Read the model definition and answer for the solid it produces. Units are mm, in the model's axes. Face numbers are marked on the shaded views. A direction names the side the tool comes from. Coordinates: 2 decimals unless noted, no trailing zeros. Loops run counter-clockwise (first coordinate to the right, second up) from the corner with the lowest first, then second, coordinate; pieces in that order, holes last. Notation, with made-up numbers: (25, 86.5) -> (41, 86.5) arc R23 cw to (41, 104.5) -> close; hole circle Ø4 at (45.5, 65). An arc over 180 degrees is marked (long way). Answer in a Markdown table with one row per item.
```python
from build123d import *

# Parameters (mm, degrees)
F0_W           = 60
F0_H           = 15
F1_DEPTH       = 7.1374
F3_D           = 3.4544
F4_D           = 4.5
F4_CBORE_D     = 7
F4_CBORE_DEPTH = 4.2
F5_SIZE        = 0.762


with BuildPart() as f1:
    # F0 (on Top) → F1 (new body)
    with BuildSketch(Plane.XY):
        Rectangle(F0_W, F0_H)
    extrude(amount=F1_DEPTH)

    # F3 (through all)
    with Locations(Plane.XY.offset(7.1374)):
        with Locations((-15, 1.76), (15, 1.76)):
            Hole(F3_D / 2)

    # F4 (through all)
    with Locations(Plane.XY.offset(7.1374)):
        with Locations((-15, -4.24), (15, -4.24)):
            CounterBoreHole(F4_D / 2, F4_CBORE_D / 2, F4_CBORE_DEPTH)

    # F5
    f5_edges = [f1.edges().sort_by_distance(p)[0] for p in [
        (0, -7.5, 7.1374),
        (-30, 0, 7.1374),
        (0, 7.5, 7.1374),
        (30, 0, 7.1374),
        (30, -7.5, 3.5687),
        (30, 7.5, 3.5687),
        (30, 0, 0),
        (0, 7.5, 0),
        (-30, 7.5, 3.5687),
        (0, -7.5, 0),
        (-30, -7.5, 3.5687),
        (-30, 0, 0),
        (23.136867, -7.5, 7.1374),
        (-23.136867, -7.5, 7.1374),
    ]]
    chamfer(f5_edges, length=F5_SIZE)


solid = f1.part
```
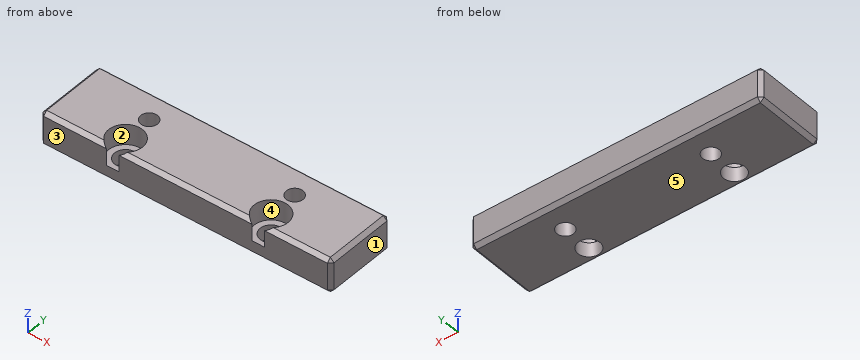
1. A cutting plane is placed at C-C on z = 1.5. Give the vertices of the cut face in (x, y).
A:
| item | result |
|---|---|
| outline | (-30, -6.74) -> (-29.24, -7.5) -> (29.24, -7.5) -> (30, -6.74) -> (30, 6.74) -> (29.24, 7.5) -> (-29.24, 7.5) -> (-30, 6.74) -> close; hole circle Ø4.5 at (-15, -4.24); hole circle Ø3.45 at (-15, 1.76); hole circle Ø4.5 at (15, -4.24); hole circle Ø3.45 at (15, 1.76) |
2. A tool of negligible diameter and unlimited length cuts with its end or side. For the marked faces 4 and 5, from which of +Z, -Z, +X, -X, +Y, -Y can it reach the whole face along a straight path? Write none if from no direction.
A:
| item | result |
|---|---|
| face 4 | +Z |
| face 5 | -Z, +X, -X, +Y, -Y |
3. A cutting plane is placed at B-B on y = 1.76. Give the vertices of the cut face in (x, z).
A:
| item | result |
|---|---|
| outline | (-30, 0.76) -> (-29.24, 0) -> (-16.73, 0) -> (-16.73, 7.14) -> (-29.24, 7.14) -> (-30, 6.38) -> close; (-13.27, 0) -> (13.27, 0) -> (13.27, 7.14) -> (-13.27, 7.14) -> close; (16.73, 0) -> (29.24, 0) -> (30, 0.76) -> (30, 6.38) -> (29.24, 7.14) -> (16.73, 7.14) -> close |
4. Given pin 1 Ø6.5 at (x, y) = (15, -4.24) entering from +Z, flat-ended and moving along its own axis, determine where the tip first touches the part or whether it passes through.
A:
| item | result |
|---|---|
| pin 1 | stops at z = 2.94 |
5. A cutting plane is placed at D-D on z = 3.75. Give the vertices of the cut face in (x, y), and give its area (3 significant figures).
A:
| item | result |
|---|---|
| outline | (-30, -6.74) -> (-29.24, -7.5) -> (-16.27, -7.5) arc R3.5 cw (long way) to (-13.73, -7.5) -> (13.73, -7.5) arc R3.5 cw (long way) to (16.27, -7.5) -> (29.24, -7.5) -> (30, -6.74) -> (30, 6.74) -> (29.24, 7.5) -> (-29.24, 7.5) -> (-30, 6.74) -> close; hole circle Ø3.45 at (-15, 1.76); hole circle Ø3.45 at (15, 1.76) |
| area | 804 mm2 |
6. Find the intervals of material crossed by probe 1 along X at (y, z) = (-4.25, 1.5); probe 2 along X at (y, z) = (-4.24, 4.6); probe 3 along Y at (x, z) = (15, 4.5), in increasing order.
A:
| item | result |
|---|---|
| probe 1 | x = -30 to -17.25, -12.75 to 12.75, 17.25 to 30 |
| probe 2 | x = -30 to -18.5, -11.5 to 11.5, 18.5 to 30 |
| probe 3 | y = -0.74 to 0.03, 3.49 to 7.5 |
7. A cutting plane is placed at A-A on x = 15. Give the vertices of the cut face in (y, z).
A:
| item | result |
|---|---|
| outline | (-7.5, 0.76) -> (-6.74, 0) -> (-6.49, 0) -> (-6.49, 2.94) -> (-7.5, 2.94) -> close; (-1.99, 0) -> (0.03, 0) -> (0.03, 7.14) -> (-0.74, 7.14) -> (-0.74, 2.94) -> (-1.99, 2.94) -> close; (3.49, 0) -> (6.74, 0) -> (7.5, 0.76) -> (7.5, 6.38) -> (6.74, 7.14) -> (3.49, 7.14) -> close |
8. The mould has two halves that part along X. Classify the marked faces 1, 2 and 3: pulls with the +X half, pulls with the -X half, needs draft (parallel to the pull), parting line crosses it, or undercut.
A:
| item | result |
|---|---|
| face 1 | pulls with the +X half |
| face 2 | undercut |
| face 3 | needs draft |
